```python
from build123d import *

# Parameters (mm, degrees)
F1_DEPTH = 25.4


with BuildPart() as f1:
    # F0 (on Front) → F1 (new body)
    with BuildSketch(Plane.XZ):
        Polygon((-22.947412, -12.524042), (-22.947412, -1.48623), (-57.528757, -1.48623), (-57.525477, -12.531252), align=None)
        Polygon((71.822926, 0), (30.506756, 0), (30.506756, -12.524042), (30.506756, -12.528093), (71.822926, -12.528093), align=None)
        Polygon((30.506756, 9.551582), (-22.947412, 9.551582), (-22.947412, -1.48623), (-22.947412, -12.524042), (30.506756, -12.524042), (30.506756, 0), align=None)
    extrude(amount=F1_DEPTH)


solid = f1.part
```
Source: CAD feature listing. Evaluate the final solid. Frame: model axes, mm. A direction names the side the tool comes from. Coordinates: 2 decimals unless noted, no trailing zeros. Write each loop counter-clockwise with the first axis right and the second up, starting at its lowest first coordinate (ties: lowest second). Pieces come first, ordered by that corner, then holes. Notation, with made-up numbers: (6, -37.75) - (10, -37.75) arc R11 ccw to (10, -19.75) - close; hole circle Ø10 at (49, 32.25). An arc over 180 degrees is marked (long way). Answer as a JSON object with one key per item and string values.
Q1. Set-up query: faces 1 (the flat face through (51, -13, 0)), 2 (the flat face through (4, -13, 9.552)), 3 (the flat face through (-22.947, -13, 4)). Return all of +Z, -Z, +X, -X, +Y, -Y with unobstructed straight access to the full face (end or side cutting, diameter ignored); none if empty.
Ans:
{"face 1": "+Z, +X, +Y, -Y", "face 2": "+Z, +X, -X, +Y, -Y", "face 3": "+Z, -X, +Y, -Y"}
Q2. Section query C-C, the plane z = 3.75. Output: boundary loops of the cut face in (x, y).
Ans:
{"outline": "(-22.95, -25.4) - (30.51, -25.4) - (30.51, 0) - (-22.95, 0) - close"}
Q3. First-contact query: pin 1 Ø12.5 at (x, y) = (54.5, -14.5) entering from -Z; pin 2 Ø6 at (y, z) = (-6.5, -10.5) entering from -X; pin 3 Ø12.5 at (x, y) = (56, -9) entering from +Z; pin 4 Ø1 at (y, z) = (-12.5, 6) entering from +X. Flat tips, straight axial feed; report the tip coordinate or a pass-through.
Ans:
{"pin 1": "stops at z = -12.53", "pin 2": "stops at x = -57.53", "pin 3": "stops at z = 0", "pin 4": "stops at x = 30.51"}
Q4. Material intervals for line 1 (X direction, y = -2.25, z = 2); line 2 (Z direction, x = -48.5, y = -4.75); line 3 (X direction, y = -17.5, z = -0.25), sorted ascending. Write a range as [from, to].
Ans:
{"line 1": "x = [-22.95, 30.51]", "line 2": "z = [-12.53, -1.49]", "line 3": "x = [-22.95, 71.82]"}
Q5. Section query B-B, the plane x = 55.5. Output: boundary loops of the cut face in (y, z), plus the area to 3 significant figures.
Ans:
{"outline": "(-25.4, -12.53) - (0, -12.53) - (0, 0) - (-25.4, 0) - close", "area": "318 mm2"}
